The listing builds one solid part. Answer for the finished solid, in the listing's coordinates (mm). Face numbers are marked on the shaded views. Give positions to 0.01 mm unless a question says otherwise; leave off trailing zeros. Write each loop counter-clockwise with the first axis right and the second up, starting at its lowest first coordinate (ties: lowest second). Pieces come first, ordered by that corner, then holes.
```python
from build123d import *

# Parameters (mm, degrees)
F1_DEPTH = 30
F2_R     = 13
F3_DEPTH = 30
F5_R     = 5
F6_DEPTH = 25


with BuildPart() as f1:
    # F0 (on Right) → F1 (new body, symmetric)
    with BuildSketch(Plane.YZ):
        Polygon((48, 40), (-48, -40), (48, -40), align=None)
    extrude(amount=F1_DEPTH, both=True)

    # F2 (on face) → F3 (cut)
    with BuildSketch(Plane(origin=(0, 48, 0), x_dir=(-1, 0, 0), z_dir=(0, 1, 0))):
        with Locations((0, -10)):
            Circle(F2_R)
    extrude(amount=-F3_DEPTH, mode=Mode.SUBTRACT)

    # F5 (on offset) → F6 (cut)
    with BuildSketch(Plane(origin=(0, 12.803688, -15.364426), x_dir=(1, 0, 0), z_dir=(0, -0.640184, 0.768221))):
        with Locations((20, -22.481997)):
            Circle(F5_R)
        with Locations((20, 37.518003)):
            Circle(F5_R)
        with Locations((-20, -22.481997)):
            Circle(F5_R)
        with Locations((-20, 37.518003)):
            Circle(F5_R)
    extrude(amount=-F6_DEPTH, mode=Mode.SUBTRACT)


solid = f1.part
```
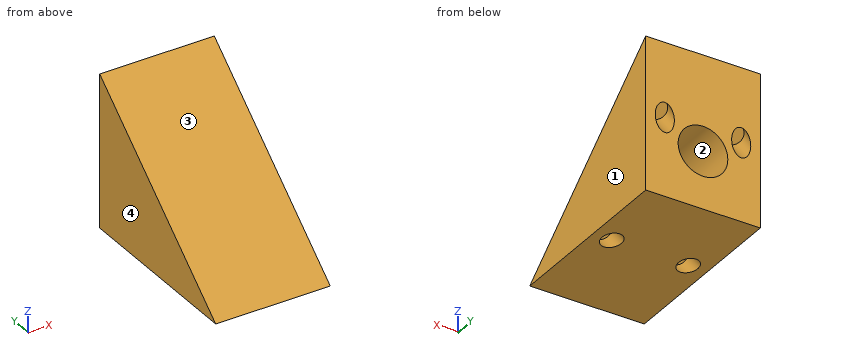
Item 1: A cutting plane is placed at C-C, the plane y = 15. Give the vertices of the cut face in (x, z), plus the area to 3 significant figures.
Conclusion:
outline: (-30, -40) - (30, -40) - (30, 12.5) - (-30, 12.5) - close
area: 3,150 mm2
Item 2: Each of these flat-tipped pins is pushed along its axis until it touches: P1, Ø5, axis at x = 0, y = -5.5, coming from the +Z side; P2, Ø21, axis at x = 5.5, z = -10, coming from the +Y side; P3, Ø21, axis at x = 0, z = -10, coming from the +Y side; P4, Ø8, axis at x = 11.5, y = -30.5, coming from the +Z side. Where does it stop, or does it pass through?
Conclusion:
P1: stops at z = -2.5
P2: stops at y = 48
P3: stops at y = 18
P4: stops at z = -22.08
Item 3: A cutting plane is placed at A-A, the plane x = 0. Give the vertices of the cut face in (y, z), plus the area to 3 significant figures.
Conclusion:
outline: (-48, -40) - (48, -40) - (48, -23) - (18, -23) - (18, 3) - (48, 3) - (48, 40) - close
area: 3,060 mm2
Item 4: Determine the mould class of the marked faces 1, 2, 3 and 4 for opening direction X: pulls with the +X half, pulls with the -X half, needs draft (parallel to the pull), parting line crosses it, or undercut.
Conclusion:
face 1: pulls with the +X half
face 2: undercut
face 3: needs draft
face 4: pulls with the -X half
Item 5: Consider probe 1 along Z at (x, y) = (0, 36); probe 2 along Z at (x, y) = (0, 32); probe 3 along Y at (x, z) = (18, -27). Determine where each line is inside the solid, lowest interval first.
Conclusion:
probe 1: z = -40 to -23, 3 to 30
probe 2: z = -40 to -23, 3 to 26.67
probe 3: y = -32.4 to -1.16, -0.8 to 48
Item 6: A cutting plane is placed at D-D, the plane x = -21. Give the vertices of the cut face in (y, z).
Conclusion:
outline: (-48, -40) - (-2.31, -40) - (-8.23, -32.89) - (-0.7, -26.62) - (10.45, -40) - (48, -40) - (48, -6.65) - (37.86, 5.52) - (45.39, 11.79) - (48, 8.66) - (48, 40) - close
Item 7: A cutting plane is placed at B-B, the plane z = -10. Give the vertices of the cut face in (x, y), plus the area to 3 significant figures.
Conclusion:
outline: (-30, -12) - (30, -12) - (30, 48) - (13, 48) - (13, 18) - (-13, 18) - (-13, 48) - (-30, 48) - close
area: 2,820 mm2
